Geometry: final body of the model. Coordinates: model frame, mm. Face numbers are marked on the shaded views. A direction names the side the tool comes from. Round coordinates to 2 decimals unless told otherwise and drop trailing zeros. Answer in a Markdown table with one row per item.
```python
from build123d import *

# Parameters (mm, degrees)
SKETCH1_W           = 7.9375
SKETCH1_H           = 7.9375
BOSS_EXTRUDE1_DEPTH = 57.15
SKETCH2_OUTSIDE_W   = 21.586
SKETCH2_OUTSIDE_H   = 21.586
CUT_EXTRUDE1_DEPTH  = 12.7
FILLET2_R           = 2.54
CUT_EXTRUDE2_DEPTH  = 58.834914911
CUT_EXTRUDE3_DEPTH  = 1.524
FILLET3_R           = 1.524


with BuildPart() as part:
    # Sketch1 → Boss-Extrude1 (new body)
    with BuildSketch(Plane.XY):
        Rectangle(SKETCH1_W, SKETCH1_H)
    extrude(amount=BOSS_EXTRUDE1_DEPTH)

    # Sketch2 outside → Cut-Extrude1 (cut)
    with BuildSketch(Plane.XY.offset(57.15)):
        Rectangle(SKETCH2_OUTSIDE_W, SKETCH2_OUTSIDE_H)
        Polygon((-3.96875, 1.841903285), (3.96875, 3.96875), (3.274308733, -3.96875), (-3.96875, -3.96875), align=None, mode=Mode.SUBTRACT)
    extrude(amount=-CUT_EXTRUDE1_DEPTH, mode=Mode.SUBTRACT)

    # Fillet2
    # the kernel refuses this fillet: 2.54 mm, written as the material it adds along each edge
    with BuildSketch(Plane(origin=(4.522188966, 10.294586333, 44.45), x_dir=(0.9961946980917462, -0.08715574274765137, 0), z_dir=(-0.08715574274765137, -0.9961946980917462, 0))) as fillet2_piece_1_section:
        with BuildLine():
            CenterArc((FILLET2_R, FILLET2_R), FILLET2_R, 180, 90)
            Line((0, FILLET2_R), (0, 0))
            Line((0, 0), (FILLET2_R, 0))
        make_face()
    fillet2_piece_1 = extrude(amount=20.667819961, mode=Mode.PRIVATE)
    fillet2_piece_1 = split(fillet2_piece_1, bisect_by=Plane(origin=(3.717682753, -3.96875, 45.282950751), z_dir=(0, 1, 0)), keep=Keep.TOP, mode=Mode.PRIVATE)
    fillet2_piece_1 = split(fillet2_piece_1, bisect_by=Plane(origin=(3.96875, -1.099038231, 45.282950751), z_dir=(-1, 0, 0)), keep=Keep.TOP, mode=Mode.PRIVATE)
    add(fillet2_piece_1)

    # Sketch3 → Cut-Extrude2 (cut, through all)
    with BuildSketch(Plane(origin=(3.96875, 0, 0), x_dir=(0, 0, -1), z_dir=(1, 0, 0))):
        Polygon((-57.15, 3.96875), (-55.750404591, -3.96875), (-57.15, -3.96875), align=None)
    extrude(amount=-CUT_EXTRUDE2_DEPTH, mode=Mode.SUBTRACT)

    # Sketch4 → Cut-Extrude3 (cut)
    with BuildSketch(Plane(origin=(-0.726331661, 2.710706661, 0), x_dir=(0.96592582628907, 0.2588190451025147, 0), z_dir=(-0.25881904510251463, 0.9659258262890699, 0))):
        Polygon((-3.356798474, -44.45), (-5.976622114, -44.45), (-5.976622114, -56.911870861), (-0.35721527, -56.911870861), (-3.356798474, -56.77497954), align=None)
        with BuildLine():
            Line((4.860706208, -44.45), (-3.356798474, -44.45))
            Line((-3.356798474, -44.45), (-3.356798474, -56.77497954))
            Line((-3.356798474, -56.77497954), (-0.35721527, -56.911870861))
            Line((-0.35721527, -56.911870861), (-0.35721527, -51.706707489))
            ThreePointArc((-0.35721527, -51.706707489), (0.386733506, -49.910656265), (2.18278473, -49.166707489))
            Line((2.18278473, -49.166707489), (4.860706208, -49.166707489))
            Line((4.860706208, -49.166707489), (4.860706208, -46.989995764))
            Line((4.860706208, -46.989995764), (4.860706208, -44.45))
        make_face()
        Polygon((8.895382264, -44.45), (4.860706208, -44.45), (4.860706208, -46.989995764), (4.860706208, -49.166707489), (4.860706208, -57.15), (8.895382264, -57.15), align=None)
    extrude(amount=-CUT_EXTRUDE3_DEPTH, mode=Mode.SUBTRACT)

    # Fillet3
    fillet3_edges = [part.edges().sort_by_distance(p)[0] for p in [
        (0, 1.327565744, 44.45),
    ]]
    fillet(fillet3_edges, radius=FILLET3_R)


solid = part.part
```
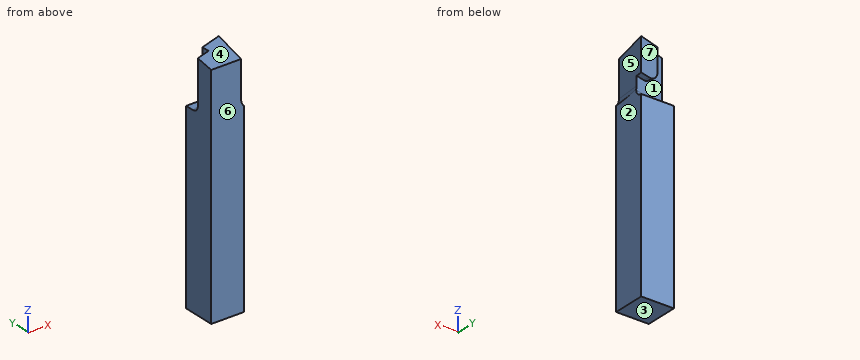
Item 1: Mould query, pull axis Z, two halves, no side actions, for the marked faces 1, 2, 3 and 4. Classes: released by +Z, released by -Z, zero draft, split by the parting line, or undercut.
Ans:
| item | result |
|---|---|
| face 1 | undercut |
| face 2 | zero draft |
| face 3 | released by -Z |
| face 4 | released by +Z |
Item 2: Set-up query: the marked faces 5, 6 and 7. Return all of +Z, -Z, +X, -X, +Y, -Y with unobstructed straight access to the full face (end or side cutting, diameter ignored); none if empty.
Ans:
| item | result |
|---|---|
| face 5 | +Z, +X, -Y |
| face 6 | +Z, -Z, +X, -X, -Y |
| face 7 | +Z, -X, +Y |
Item 3: Ray query, L1, parallel to Z at x = 0, y = 2.75; L2, parallel to Z at x = 1.25, y = 2; L3, parallel to Z at x = 1, y = 1. Return the intervals inside material, ascending.
Ans:
| item | result |
|---|---|
| L1 | 0 to 44.46, 49.64 to 56.94 |
| L2 | 0 to 45.03, 49.21 to 56.8 |
| L3 | 0 to 56.63 |
Item 4: First-contact query: P1, Ø0.6, axis at x = -1.5, y = 3, coming from the +Z side. Flat tip, straight axial feed; report the tip coordinate or a pass-through.
Ans:
| item | result |
|---|---|
| P1 | z = 44.45 |
